from build123d import *

# Parameters (mm, degrees)
SKETCH2_W           = 7.02
SKETCH2_H           = 4.25
BOSS_EXTRUDE1_DEPTH = 7.875
SKETCH4_W           = 1
SKETCH4_H           = 1
LPATTERN1_COUNT     = 4
LPATTERN1_PITCH     = 3.833333333


with BuildPart() as part:
    # Sketch2 → Boss-Extrude1 (new, symmetric)
    with BuildSketch(Plane(origin=(0, 0, 0), x_dir=(0, 0, -1), z_dir=(1, 0, 0))):
        with Locations((-3.51, -2.125)):
            Rectangle(SKETCH2_W, SKETCH2_H)
        Polygon((0, 3.95), (0, 0), (0, -2.125), (1.12, -2.125), (1.12, 3.95), (1.72, 3.95), (1.46, 6.25), (0.26, 6.25), align=None)
    extrude(amount=BOSS_EXTRUDE1_DEPTH, both=True)

    # Sweep1: sweep along a path in Sketch3
    with BuildLine(Plane(origin=(5.75, 0, 0), x_dir=(0, 0, -1), z_dir=(1, 0, 0))) as sweep1_path:
        Line((-2.03, 6.05), (-2.03, -1.85))
        ThreePointArc((-2.03, -1.85), (-2.615786438, -3.264213562), (-4.03, -3.85))
        Line((-4.03, -3.85), (-9.58, -3.85))
    # Sketch4 → Sweep1 (sweep)
    with BuildSketch(Plane(origin=(0, 6.05, 0), x_dir=(1, 0, 0), z_dir=(0, 1, 0))):
        with Locations((5.75, -2.03)):
            Rectangle(SKETCH4_W, SKETCH4_H)
    sweep1 = sweep(path=sweep1_path.line)

    # LPattern1: Sweep1 ×4
    with Locations(*[(-i * LPATTERN1_PITCH, 0, 0) for i in range(1, LPATTERN1_COUNT)]):
        add(sweep1)


solid = part.part
Model file for the job. Use its own axes, mm. A direction names the side the tool comes from. Give positions to 0.01 mm unless a question says otherwise; leave off trailing zeros. Order: outer loops, then holes, each group sorted by start corner. A loop starts at its lowest first (then second) coordinate and runs counter-clockwise, first axis right, second up. Notation, with made-up numbers: M 42,84.5 L 65,84.5 A9 cw 65,98.5 Z; hole C 30,-36 d8. An arc over 180 degrees is marked long. Put each result on its own line as item: value. Start each with the question number.
(1) Band-saw the part on D-D on y = 5.5. Give the cut face in (x, z) (3 decimals).
(2) Band-saw the part on C-C on z = 2. Give the cut face in (x, y) (3 decimals).
(3) Drill centre lines: L1, parallel to X at y = 2.5, z = 2.25; L2, parallel to Z at x = 1.5, y = 2; L3, parallel to Z at x = 0.25, y = -1.5. Where is each one in solid material? Low to high. Write a range as [from, to].
(4) Pin check, flat tips, straight feed: pin 1 Ø0.8 at (x, y) = (-2, 4.5) entering from -Z; pin 2 Ø1.1 at (x, z) = (-6, 8) entering from +Y; pin 3 Ø2 at (x, y) = (3, -2) entering from +Z. Stop position of each tip, or through.
(5) Tool access for faces 1 (the face through (-5.25, -4, 8)), 2 (the face through (1.417, 3, 2)), 3 (the face through (6, 6.05, 2)): list every direction of +Z, -Z, +X, -X, +Y, -Y with a clear straight run to the whole face (end or side of a thin tool).
(6) Band-saw the part on A-A on y = 2. Give the cut face in (x, z) (3 decimals).
(7) Band-saw the part on B-B on x = 3.5. Give the cut face in (y, z) (3 decimals).
(8) Pull direction Z, two halves, no side cores. Call faces 4 (the face through (2, 3, 1.53)), 5 (the face through (2, 3, 2.53)), 6 (the face through (-6, -3.35, 8)): released by +Z, released by -Z, zero draft, split by the parting line, or undercut.
Results below:
1. outline: M -7.875,-1.545 L 7.875,-1.545 L 7.875,-0.175 L -7.875,-0.175 Z; M -6.25,1.53 L -5.25,1.53 L -5.25,2.53 L -6.25,2.53 Z; M -2.417,1.53 L -1.417,1.53 L -1.417,2.53 L -2.417,2.53 Z; M 1.417,1.53 L 2.417,1.53 L 2.417,2.53 L 1.417,2.53 Z; M 5.25,1.53 L 6.25,1.53 L 6.25,2.53 L 5.25,2.53 Z
2. outline: M -7.875,-4.25 L 7.875,-4.25 L 7.875,0 L 6.25,0 L 6.25,6.05 L 5.25,6.05 L 5.25,0 L 2.417,0 L 2.417,6.05 L 1.417,6.05 L 1.417,0 L -1.417,0 L -1.417,6.05 L -2.417,6.05 L -2.417,0 L -5.25,0 L -5.25,6.05 L -6.25,6.05 L -6.25,0 L -7.875,0 Z
3. L1: x = [-6.25, -5.25], [-2.42, -1.42], [1.42, 2.42], [5.25, 6.25]
3. L2: z = [-1.12, 0], [1.53, 2.53]
3. L3: z = [-1.12, 7.02]
4. pin 1: stops at z = -1.7
4. pin 2: stops at y = -3.35
4. pin 3: stops at z = 7.02
5. face 1: +Z, -Y
5. face 2: +Z, +Y
5. face 3: +Z, +X, -X, +Y
6. outline: M -7.875,-1.12 L 7.875,-1.12 L 7.875,0 L -7.875,0 Z; M -6.25,1.53 L -5.25,1.53 L -5.25,2.53 L -6.25,2.53 Z; M -2.417,1.53 L -1.417,1.53 L -1.417,2.53 L -2.417,2.53 Z; M 1.417,1.53 L 2.417,1.53 L 2.417,2.53 L 1.417,2.53 Z; M 5.25,1.53 L 6.25,1.53 L 6.25,2.53 L 5.25,2.53 Z
7. outline: M -4.25,0 L -2.125,0 L -2.125,-1.12 L 3.95,-1.12 L 3.95,-1.72 L 6.25,-1.46 L 6.25,-0.26 L 3.95,0 L 0,0 L 0,7.02 L -4.25,7.02 Z
8. face 4: undercut
8. face 5: released by +Z
8. face 6: zero draft
